Read the model definition and answer for the solid it produces. Units are mm, in the model's axes. Face numbers are marked on the shaded views. A direction names the side the tool comes from. Round coordinates to 2 decimals unless told otherwise and drop trailing zeros. Order: outer loops, then holes, each group sorted by start corner. A loop starts at its lowest first (then second) coordinate and runs counter-clockwise, first axis right, second up. Notation, with made-up numbers: (-8.5, 0.5) -> (33.5, 0.5) arc R18 cw to (33.5, 20.5) -> close; hole circle Ø11 at (7, 63.5). An arc over 180 degrees is marked (long way). Answer as a JSON object with one key per item and string values. Group by question number.
Item 1: For the marked faces 1 and 2, determine the directions among +Z, -Z, +X, -X, +Y, -Y from which every point of the face is accessible in a straight line to the end or side of a thin tool.
Item 2: Section A-A, the plane x = 8.5 is taken. Write down the section's boundary in (y, z).
Item 3: Section C-C, the plane y = 6.75 is taken. Write down the section's boundary in (x, z).
Item 4: Consider probe 1 along Z at (x, y) = (31, 3.75); probe 2 along Y at (x, z) = (9.5, 4); probe 3 along Y at (x, z) = (31, 19.5). Determine where each line is inside the solid, lowest interval first. Write a range as from..to.
Item 5: Section B-B, the plane z = 11.5 is taken. Write down the section's boundary in (x, y), plus the area to 3 significant figures.
Item 6: Given P1, Ø13, axis at x = 11, z = 16.5, coming from the +Y side; P2, Ø1.5, axis at y = 0, z = 11.5, coming from the -X side; P3, Ø1.5, axis at y = 4, z = 38, coming from the +X side; P4, Ø6, axis at y = 6, z = 25, coming from the +X side, each flat-ended and moving along its own axis, determine where each tip first touches the part or whether it passes through.
from build123d import *

# Parameters (mm, degrees)
EXTRUDE_1_DEPTH = 50
M3X0_5_1_D      = 2.5
M3X0_5_1_DEPTH  = 8.5
M3X0_5_1_TIP    = 0.751075774


with BuildPart() as part:
    # ｽｹｯﾁ1 → ﾎﾞｽ - 押し出し1 (new body)
    with BuildSketch(Plane.XY):
        Polygon((0, 0), (25.772059531, 0), (36.705091427, 9.173903032), (37.990666647, 7.641814145), (26.5, -2), (0, -2), align=None)
    extrude(amount=EXTRUDE_1_DEPTH)

    # M3x0.5 ねじ穴1
    with Locations(Plane(origin=(30.751348412, 4.178119463, 25), x_dir=(0.766044443, 0.64278761, 0), z_dir=(-0.64278761, 0.766044443, 0))):
        with Locations((0, 0)):
            Hole(M3X0_5_1_D / 2, depth=M3X0_5_1_DEPTH)
            with Locations((0, 0, -(M3X0_5_1_DEPTH + M3X0_5_1_TIP / 2))):  # 118° drill point
                Cone(0, M3X0_5_1_D / 2, M3X0_5_1_TIP, mode=Mode.SUBTRACT)


solid = part.part
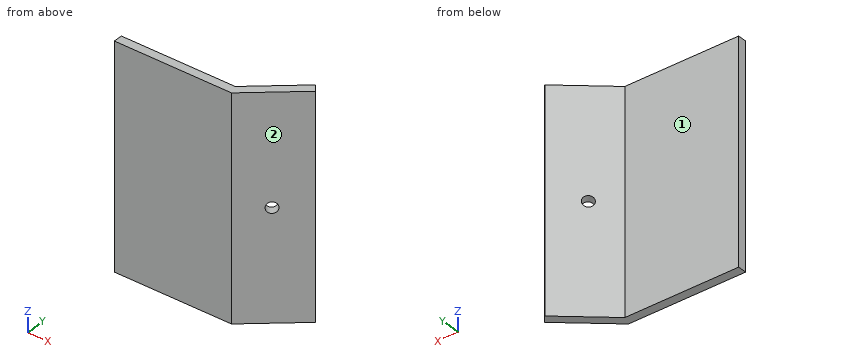
Values found:
{
 "1": {"face 1": "+Z, -Z, -X, +Y", "face 2": "+Z, -Z, +X, -Y"},
 "2": {"outline": "(-2, 0) -> (0, 0) -> (0, 50) -> (-2, 50) -> close"},
 "3": {"outline": "(33.82, 0) -> (36.93, 0) -> (36.93, 50) -> (33.82, 50) -> close"},
 "4": {"probe 1": "0..23.75, 26.25..50", "probe 2": "-2..0", "probe 3": "1.78..4.39"},
 "5": {"outline": "(0, -2) -> (26.5, -2) -> (37.99, 7.64) -> (36.71, 9.17) -> (25.77, 0) -> (0, 0) -> close", "area": "81.5 mm2"},
 "6": {"P1": "y = 0", "P2": "x = 0", "P3": "x = 34.54", "P4": "x = 37.99"}
}
